Check sheet for the modelled part. Datum: model origin and axes. Units: mm. Face numbers are marked on the shaded views. A direction names the side the tool comes from. Round coordinates to 2 decimals unless told otherwise and drop trailing zeros. Order: outer loops, then holes, each group sorted by start corner. A loop starts at its lowest first (then second) coordinate and runs counter-clockwise, first axis right, second up. Notation, with made-up numbers: (-4.75, -25) -> (40.25, -25) arc R30 ccw to (40.25, -1) -> close; hole circle Ø2 at (5, 60.25). An arc over 180 degrees is marked (long way). Answer in a Markdown table with one row per item.
```python
from build123d import *

# Parameters (mm, degrees)
F0_W      = 10
F0_H      = 100
F1_DEPTH  = 10
F0_W_2    = 20.8
F2_DEPTH  = 5
F3_W      = 40.8
F3_H      = 5
F4_DEPTH  = 15
F5_W      = 40.8
F5_H      = 10
F6_DEPTH  = 5
F7_W      = 8
F7_H      = 20
F8_DEPTH  = 22
F9_R      = 3.5
F10_DEPTH = 33.401
F11_DEPTH = 5
F12_R     = 9.99999
F13_R     = 4.99999
F14_R     = 2
F15_W     = 100
F15_H     = 3.5
F16_DEPTH = 5
F17_W     = 100
F17_H     = 3.5
F18_DEPTH = 5
F19_DEPTH = 2


# Not quite as in the source:
# - a fillet or chamfer is up to 0.001 mm smaller than in the source, because OpenCascade refuses the exact size


with BuildPart() as f1:
    # F0 (on Top) → F1 (new body)
    with BuildSketch(Plane.XY):
        with Locations((-15.4, 0)):
            Rectangle(F0_W, F0_H)
        Polygon((-10.4, 50), (10.4, 50), (20.4, 50), (20.4, 60), (-20.4, 60), (-20.4, 50), align=None)
        with Locations((15.4, 0)):
            Rectangle(F0_W, F0_H)
    extrude(amount=F1_DEPTH)

    # F0 (on Top) → F2 (join)
    with BuildSketch(Plane.XY):
        Rectangle(F0_W_2, F0_H)
        with BuildLine():
            Line((3.5661098082, 10), (3.5661098082, -40))
            ThreePointArc((3.5661098082, -40), (0, -43.5661098082), (-3.5661098082, -40))
            Line((-3.5661098082, -40), (-3.5661098082, 10))
            ThreePointArc((-3.5661098082, 10), (0, 13.5661098082), (3.5661098082, 10))
        make_face(mode=Mode.SUBTRACT)
    extrude(amount=F2_DEPTH)

    # F3 (on face) → F4 (join)
    with BuildSketch(Plane.XY.offset(10)):
        with Locations((0, 57.5)):
            Rectangle(F3_W, F3_H)
    extrude(amount=F4_DEPTH)

    # F5 (on face) → F6 (join)
    with BuildSketch(Plane.XY.offset(25)):
        with Locations((0, 55)):
            Rectangle(F5_W, F5_H)
    extrude(amount=F6_DEPTH)

    # F7 (on face) → F8 (join)
    with BuildSketch(Plane(origin=(0, 0, 0), x_dir=(1, 0, 0), z_dir=(0, 0, -1))):
        with Locations((9, -42.3806495965)):
            Rectangle(F7_W, F7_H)
        with Locations((-9, -42.3806495965)):
            Rectangle(F7_W, F7_H)
    extrude(amount=F8_DEPTH)

    # F9 (on face) → F10 (cut, through all)
    with BuildSketch(Plane(origin=(-13, 0, 0), x_dir=(0, -1, 0), z_dir=(-1, 0, 0))):
        with Locations((-42.3806495965, -13)):
            Circle(F9_R)
    extrude(amount=-F10_DEPTH, mode=Mode.SUBTRACT)

    # F9 (on face) → F11 (cut)
    with BuildSketch(Plane(origin=(-13, 0, 0), x_dir=(0, -1, 0), z_dir=(-1, 0, 0))):
        Polygon((-39.0320180352, -7.2), (-45.7292811578, -7.2), (-49.0779127191, -13), (-45.7292811578, -18.8), (-39.0320180352, -18.8), (-35.6833864739, -13), align=None)
        with Locations((-42.3806495965, -13)):
            Circle(F9_R, mode=Mode.SUBTRACT)
    extrude(amount=-F11_DEPTH, mode=Mode.SUBTRACT)

    # F12 (radius 10 in the source; OpenCascade refuses exactly that, so slightly less here)
    f12_edges = [f1.edges().sort_by_distance(p)[0] for p in [
        (-9, 52.38065, -22),
        (9, 52.38065, -22),
        (9, 32.38065, -22),
        (-9, 32.38065, -22),
    ]]
    fillet(f12_edges, radius=F12_R)

    # F13 (radius 5 in the source; OpenCascade refuses exactly that, so slightly less here)
    f13_edges = [f1.edges().sort_by_distance(p)[0] for p in [
        (-20.4, 50, 27.5),
        (20.4, 50, 27.5),
        (0, 60, 30),
        (0, 60, 0),
    ]]
    fillet(f13_edges, radius=F13_R)

    # F14
    f14_edges = [f1.edges().sort_by_distance(p)[0] for p in [
        (-20.4, 55, 17.5),
        (20.4, 55, 17.5),
        (-20.4, -50, 5),
        (20.4, -50, 5),
    ]]
    fillet(f14_edges, radius=F14_R)

    # F15 (on face) → F16 (cut)
    with BuildSketch(Plane.YZ.offset(-10.4)):
        with Locations((0, 6.75)):
            Rectangle(F15_W, F15_H)
    extrude(amount=-F16_DEPTH, mode=Mode.SUBTRACT)

    # F17 (on face) → F18 (cut)
    with BuildSketch(Plane(origin=(10.4, 0, 0), x_dir=(0, -1, 0), z_dir=(-1, 0, 0))):
        with Locations((0, 6.75)):
            Rectangle(F17_W, F17_H)
    extrude(amount=-F18_DEPTH, mode=Mode.SUBTRACT)

    # F19 (cut): a face of the model
    f19_faces = [f1.faces().sort_by_distance(p)[0] for p in [
        (0, 48.9536425085, 5),
    ]]
    extrude(f19_faces, amount=-F19_DEPTH, mode=Mode.SUBTRACT)


solid = f1.part
```
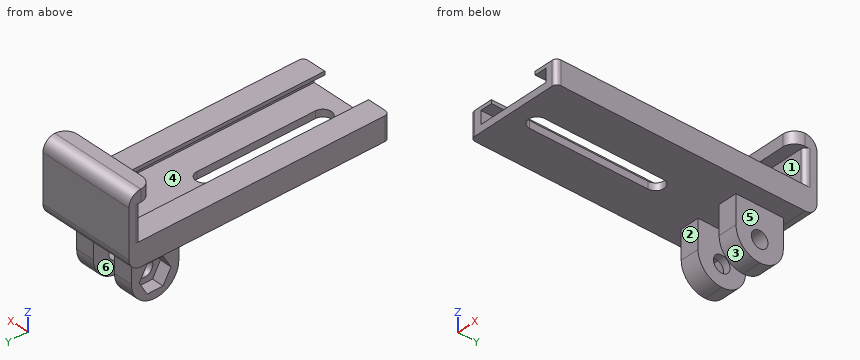
(1) Section check A-A on x = 0. Record the boundary of the cut face in (y, z).
Solutions:
| item | result |
|---|---|
| outline | (-50, 0) -> (-43.57, 0) -> (-43.57, 3) -> (-50, 3) -> close; (13.57, 0) -> (55, 0) arc R5 ccw to (60, 5) -> (60, 25) arc R5 ccw to (55, 30) -> (50, 30) -> (50, 25) -> (55, 25) -> (55, 10) -> (50, 10) -> (50, 3) -> (13.57, 3) -> close |
(2) Section check B-B on y = 12. Record the boundary of the cut face in (x, z).
Solutions:
| item | result |
|---|---|
| outline | (-20.4, 0) -> (-2.95, 0) -> (-2.95, 3) -> (-15.4, 3) -> (-15.4, 8.5) -> (-10.4, 8.5) -> (-10.4, 10) -> (-20.4, 10) -> close; (2.95, 0) -> (20.4, 0) -> (20.4, 10) -> (10.4, 10) -> (10.4, 8.5) -> (15.4, 8.5) -> (15.4, 3) -> (2.95, 3) -> close |
(3) Depth check by flat-ended pin: pin 1 Ø6 at (y, z) = (40.5, -8) entering from +X; pin 2 Ø6 at (x, z) = (-4, 8) entering from -Y; pin 3 Ø9 at (x, z) = (-8.5, -5.5) entering from +Y; pin 4 Ø5.5 at (x, z) = (-4.5, 5.5) entering from -Y. Enter the tip coordinate at first touch or a pass-through.
Solutions:
| item | result |
|---|---|
| pin 1 | x = 13 |
| pin 2 | y = 50 |
| pin 3 | y = 52.38 |
| pin 4 | y = -50 |
(4) Section check C-C on z = -14.5. Record the boundary of the cut face in (x, y).
Solutions:
| item | result |
|---|---|
| outline | (-13, 32.7) -> (-5, 32.7) -> (-5, 39.22) -> (-8, 39.22) -> (-8, 36.55) -> (-13, 36.55) -> close; (-13, 48.21) -> (-8, 48.21) -> (-8, 45.54) -> (-5, 45.54) -> (-5, 52.06) -> (-13, 52.06) -> close; (5, 32.7) -> (13, 32.7) -> (13, 39.22) -> (5, 39.22) -> close; (5, 45.54) -> (13, 45.54) -> (13, 52.06) -> (5, 52.06) -> close |
(5) Draft check along Z on the marked faces 1, 2 and 3. Enter one of: pulls with the +Z half, pulls with the -Z half, needs draft (parallel to the pull), parting line crosses it, or undercut.
Solutions:
| item | result |
|---|---|
| face 1 | undercut |
| face 2 | needs draft |
| face 3 | pulls with the -Z half |
(6) Section check D-D on z = 6.5. Record the boundary of the cut face in (x, y), plus the area to 3 significant figures.
Solutions:
| item | result |
|---|---|
| outline | (-20.4, -48) arc R2 ccw to (-18.4, -50) -> (-15.4, -50) -> (-15.4, 50) -> (15.4, 50) -> (15.4, -50) -> (18.4, -50) arc R2 ccw to (20.4, -48) -> (20.4, 60) -> (-20.4, 60) -> close |
| area | 1,410 mm^2 |
(7) Scan lines: probe 1 along Z at (x, y) = (13.5, -17); probe 2 along X at (y, z) = (50, -5); probe 3 along X at (y, z) = (40, 3.5). Record each from-to range of solid material in increasing order. Write a range as from..to.
Solutions:
| item | result |
|---|---|
| probe 1 | 0..3, 8.5..10 |
| probe 2 | -13..-5, 5..13 |
| probe 3 | -20.4..-15.4, 15.4..20.4 |
(8) Tool access check on the marked faces 4, 5 and 6. Record the directions out of +Z, -Z, +X, -X, +Y, -Y that give a thin tool (end or side, any length) a straight path to the whole face; none if there is none.
Solutions:
| item | result |
|---|---|
| face 4 | -Y |
| face 5 | -Z, +X, +Y, -Y |
| face 6 | -Z, +Y, -Y |
